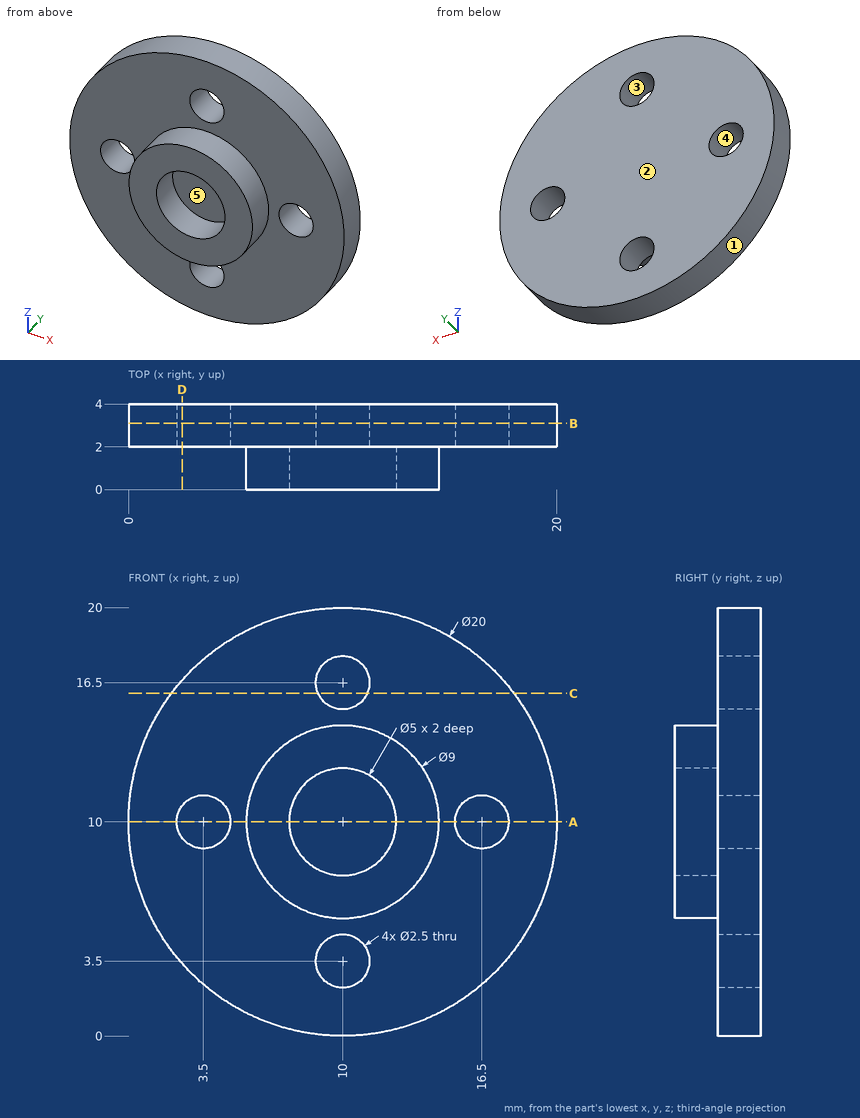
Can you work these out from the drawing? Everything is in mm from the part's minimum corner. A direction names the side the tool comes from. Round coordinates to 2 decimals unless told otherwise and drop trailing zeros. Write each loop counter-clockwise with the first axis right and the second up, starting at its lowest first coordinate (ties: lowest second). Pieces come first, ordered by that corner, then holes.
1. Will these pins go through, and if not, where does the flat tip stop? pin 1 Ø1.5 at (y, z) = (3.5, 2.5) entering from +X; pin 2 Ø2 at (x, y) = (13.5, 1.5) entering from +Z; pin 3 Ø1 at (x, y) = (16, 2.5) entering from +Z; pin 4 Ø2 at (x, z) = (16.5, 10) entering from -Y.
2. I need wall thicknesses on L1, parallel to X at y = 3.1, z = 10; L2, parallel to Y at x = 5.75, z = 1.75; L3, parallel to X at y = 2.4, z = 16.5. Which ranges of each line are inside material? Lowest first, please.
3. Suppose I cut it at B-B (y = 3.1). List the corners of the cut face in (x, z) for me, and give its area (3 significant figures).
4. Suppose I cut it at D-D (x = 2.5). List the corners of the cut face in (y, z) for me.
5. Suppose I cut it at A-A (z = 10). List the corners of the cut face in (x, y) for me, and give its area (3 significant figures).
6. For the marked faces 4 and 5, which set-ups out of +Z, -Z, +X, -X, +Y, -Y let a thin tool reach every point of the face, with its end or its side?
7. If we mould it in two halves opening along Z, with no side actions, what happens to the marked faces 1, 2 and 3? For each: released by +Z, released by -Z, zero draft, split by the parting line, or undercut.
8. Suppose I cut it at C-C (z = 16). List the corners of the cut face in (x, y) for me.
Answer sheet:
1. pin 1: stops at x = 17.38
1. pin 2: stops at z = 19.65
1. pin 3: stops at z = 18.35
1. pin 4: passes through
2. L1: x = 0 to 2.25, 4.75 to 15.25, 17.75 to 20
2. L2: y = 2 to 4
2. L3: x = 2.4 to 8.75, 11.25 to 17.6
3. outline: circle Ø20 at (10, 10); hole circle Ø2.5 at (3.5, 10); hole circle Ø2.5 at (10, 3.5); hole circle Ø2.5 at (10, 16.5); hole circle Ø2.5 at (16.5, 10)
3. area: 295 mm2
4. outline: (2, 3.39) - (4, 3.39) - (4, 9.25) - (2, 9.25) - close; (2, 10.75) - (4, 10.75) - (4, 16.61) - (2, 16.61) - close
5. outline: (0, 2) - (2.25, 2) - (2.25, 4) - (0, 4) - close; (4.75, 2) - (5.5, 2) - (5.5, 0) - (7.5, 0) - (7.5, 2) - (12.5, 2) - (12.5, 0) - (14.5, 0) - (14.5, 2) - (15.25, 2) - (15.25, 4) - (4.75, 4) - close; (17.75, 2) - (20, 2) - (20, 4) - (17.75, 4) - close
5. area: 38.0 mm2
6. face 4: +Y, -Y
6. face 5: -Y
7. face 1: split by the parting line
7. face 2: zero draft
7. face 3: undercut
8. outline: (2, 2) - (8.85, 2) - (8.85, 4) - (2, 4) - close; (11.15, 2) - (18, 2) - (18, 4) - (11.15, 4) - close
